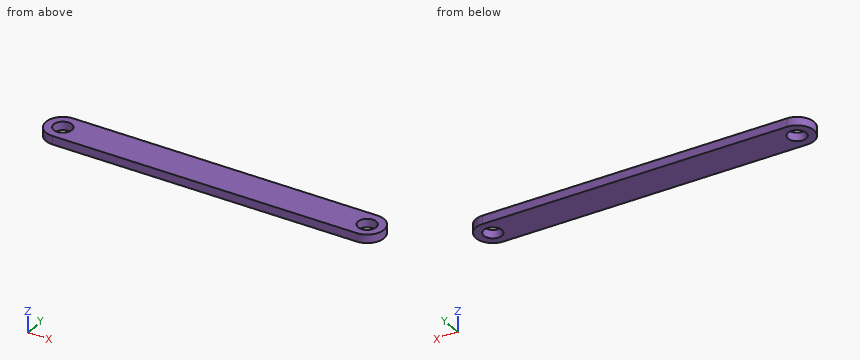
from build123d import *

# Parameters (mm, degrees)
SKETCH1_W           = 200
SKETCH1_H           = 20
BOSS_EXTRUDE1_DEPTH = 5
FILLET1_RADIUS      = 10
FILLET1_LENGTH      = 5
FILLET2_RADIUS      = 10
FILLET2_LENGTH      = 5
SKETCH2_R           = 5.4
CUT_EXTRUDE1_DEPTH  = 5


with BuildPart() as part:
    # Sketch1 → Boss-Extrude1 (new body)
    with BuildSketch(Plane.XY):
        with Locations((100, 10)):
            Rectangle(SKETCH1_W, SKETCH1_H)
    extrude(amount=BOSS_EXTRUDE1_DEPTH)

    # Fillet1: full round fillet: the end face becomes a half cylinder, R = half its width
    fillet1_face = Plane((200, 10, 2.5), x_dir=(0, 0, 1), z_dir=(1, 0, 0))  # on the end face: x along it, z out of the body
    fillet1_slab = fillet1_face.offset(-FILLET1_RADIUS / 2) * Box(FILLET1_LENGTH, 2 * FILLET1_RADIUS, FILLET1_RADIUS, mode=Mode.PRIVATE)  # the body's end, R deep
    fillet1_round = Plane((190, 10, 2.5), x_dir=(1, 0, 0), z_dir=(0, 0, 1)) * Cylinder(FILLET1_RADIUS, FILLET1_LENGTH, mode=Mode.PRIVATE)  # its axis R under the face
    add(fillet1_slab - fillet1_round, mode=Mode.SUBTRACT)

    # Fillet2: full round fillet: the end face becomes a half cylinder, R = half its width
    fillet2_face = Plane((0, 10, 2.5), x_dir=(0, 0, -1), z_dir=(-1, 0, 0))  # on the end face: x along it, z out of the body
    fillet2_slab = fillet2_face.offset(-FILLET2_RADIUS / 2) * Box(FILLET2_LENGTH, 2 * FILLET2_RADIUS, FILLET2_RADIUS, mode=Mode.PRIVATE)  # the body's end, R deep
    fillet2_round = Plane((10, 10, 2.5), x_dir=(-1, 0, 0), z_dir=(0, 0, -1)) * Cylinder(FILLET2_RADIUS, FILLET2_LENGTH, mode=Mode.PRIVATE)  # its axis R under the face
    add(fillet2_slab - fillet2_round, mode=Mode.SUBTRACT)

    # Sketch2 → Cut-Extrude1 (cut)
    with BuildSketch(Plane.XY.offset(5)):
        with Locations((10, 10)):
            Circle(SKETCH2_R)
        with Locations((190, 10)):
            Circle(SKETCH2_R)
    extrude(amount=-CUT_EXTRUDE1_DEPTH, mode=Mode.SUBTRACT)


solid = part.part
Read the model definition and answer for the solid it produces. Units are mm, in the model's axes. Round coordinates to 2 decimals unless told otherwise and drop trailing zeros. Order: outer loops, then holes, each group sorted by start corner. A loop starts at its lowest first (then second) coordinate and runs counter-clockwise, first axis right, second up.
1) Flat-ended cylindrical pins translate along their axes: pin 1 (9.5 mm diameter, centred on x = 10, y = 10, fed in from +Z); pin 2 (2 mm diameter, centred on y = 17.5, z = 0.5, fed in from -X). Find the tip coordinate at first contact, or state that the pin passes through.
2) The part is cut by section A-A on y = 10. Write down the section's boundary in (x, z).
3) The part is cut by section B-B on z = 2.6. Write down the section's boundary in (x, y), plus the area to 3 significant figures.
4) Straight lines are drawn through the part: L1, parallel to X at y = 10.25, z = 4.65; L2, parallel to X at y = 12.5, z = 2.25; L3, parallel to Y at x = 10, z = 2.75. For each, find the intervals that lie inside material, in ascending order.
5) The part is cut by section C-C on y = 18.25. Write down the section's boundary in (x, z).
6) The part is cut by section D-D on y = 2.5. Write down the section's boundary in (x, z).
Resolved:
1. pin 1: passes through
1. pin 2: stops at x = 2.4
2. outline: (0, 0) - (4.6, 0) - (4.6, 5) - (0, 5) - close; (15.4, 0) - (184.6, 0) - (184.6, 5) - (15.4, 5) - close; (195.4, 0) - (200, 0) - (200, 5) - (195.4, 5) - close
3. outline: (10, 0) - (190, 0) arc R10 ccw to (190, 20) - (10, 20) arc R10 ccw to start; hole circle Ø10.8 at (10, 10); hole circle Ø10.8 at (190, 10)
3. area: 3,730 mm2
4. L1: x = 0 to 4.61, 15.39 to 184.61, 195.39 to 200
4. L2: x = 0.32 to 5.21, 14.79 to 185.21, 194.79 to 199.68
4. L3: y = 0 to 4.6, 15.4 to 20
5. outline: (4.35, 0) - (195.65, 0) - (195.65, 5) - (4.35, 5) - close
6. outline: (3.39, 0) - (196.61, 0) - (196.61, 5) - (3.39, 5) - close
